from build123d import *

# Parameters (mm, degrees)
SZKIC1_W                    = 40
SZKIC1_H                    = 28
SZKIC1_R                    = 11
DODANIE_WYCI_GNI_CIE1_DEPTH = 10
SZKIC2_W                    = 40
SZKIC2_H                    = 28
DODANIE_WYCI_GNI_CIE2_DEPTH = 3
SFAZOWANIE1_SIZE            = 2
SZKIC3_R                    = 4.3
WYTNIJ_WYCI_GNI_CIE1_DEPTH  = 3
SZKIC4_R                    = 2
WYTNIJ_WYCI_GNI_CIE2_DEPTH  = 6
ZAOKR_GLENIE1_SIZE          = 14
ZAOKR_GLENIE1_SIZE_2        = 8
ZAOKR_GLENIE2_SIZE          = 14
ZAOKR_GLENIE2_SIZE_2        = 8
SZKIC5_R                    = 2.6
WYTNIJ_WYCI_GNI_CIE3_DEPTH  = 7


with BuildPart() as part:
    # Szkic1 → Dodanie-wyciągnięcie1 (new body)
    with BuildSketch(Plane.XY):
        Rectangle(SZKIC1_W, SZKIC1_H)
        Circle(SZKIC1_R, mode=Mode.SUBTRACT)
    extrude(amount=DODANIE_WYCI_GNI_CIE1_DEPTH)

    # Szkic2 → Dodanie-wyciągnięcie2 (add)
    with BuildSketch(Plane(origin=(0, 0, 0), x_dir=(-1, 0, 0), z_dir=(0, 0, -1))):
        Rectangle(SZKIC2_W, SZKIC2_H)
    extrude(amount=DODANIE_WYCI_GNI_CIE2_DEPTH)

    # Sfazowanie1
    sfazowanie1_edges = [part.edges().sort_by_distance(p)[0] for p in [
        (-11, 0, 0),
    ]]
    chamfer(sfazowanie1_edges, length=SFAZOWANIE1_SIZE)

    # Szkic3 → Wytnij-wyciągnięcie1 (cut)
    with BuildSketch(Plane.XY):
        Circle(SZKIC3_R)
    extrude(amount=-WYTNIJ_WYCI_GNI_CIE1_DEPTH, mode=Mode.SUBTRACT)

    # Szkic4 → Wytnij-wyciągnięcie2 (cut)
    with BuildSketch(Plane.XY.offset(10)):
        with Locations((-15, 0)):
            Circle(SZKIC4_R)
        with Locations((15, 0)):
            Circle(SZKIC4_R)
    extrude(amount=-WYTNIJ_WYCI_GNI_CIE2_DEPTH, mode=Mode.SUBTRACT)

    # Zaokrąglenie1
    # an asymmetric fillet: 14, 8 mm, written as the material it takes off along each edge
    with BuildSketch(Plane(origin=(20, -14, -38), x_dir=(-1, 0, 0), z_dir=(0, 0, 1))) as zaokr_glenie1_piece_1:
        with BuildLine():
            Bezier((ZAOKR_GLENIE1_SIZE, 0), (0, 0), (0, -ZAOKR_GLENIE1_SIZE_2), weights=[1, 0.707106781, 1])
            Line((0, -ZAOKR_GLENIE1_SIZE_2), (0, 0))
            Line((0, 0), (ZAOKR_GLENIE1_SIZE, 0))
        make_face()
    extrude(amount=83, mode=Mode.SUBTRACT)
    with BuildSketch(Plane(origin=(-20, 14, 45), x_dir=(0, -1, 0), z_dir=(0, 0, -1))) as zaokr_glenie1_piece_2:
        with BuildLine():
            Bezier((ZAOKR_GLENIE1_SIZE_2, 0), (0, 0), (0, -ZAOKR_GLENIE1_SIZE), weights=[1, 0.707106781, 1])
            Line((0, -ZAOKR_GLENIE1_SIZE), (0, 0))
            Line((0, 0), (ZAOKR_GLENIE1_SIZE_2, 0))
        make_face()
    extrude(amount=83, mode=Mode.SUBTRACT)

    # Zaokrąglenie2
    # an asymmetric fillet: 14, 8 mm, written as the material it takes off along each edge
    with BuildSketch(Plane(origin=(20, 14, -38), x_dir=(-1, 0, 0), z_dir=(0, 0, 1))) as zaokr_glenie2_piece_1:
        with BuildLine():
            Bezier((ZAOKR_GLENIE2_SIZE, 0), (0, 0), (0, ZAOKR_GLENIE2_SIZE_2), weights=[1, 0.707106781, 1])
            Line((0, ZAOKR_GLENIE2_SIZE_2), (0, 0))
            Line((0, 0), (ZAOKR_GLENIE2_SIZE, 0))
        make_face()
    extrude(amount=83, mode=Mode.SUBTRACT)
    with BuildSketch(Plane(origin=(-20, -14, 45), x_dir=(1, 0, 0), z_dir=(0, 0, -1))) as zaokr_glenie2_piece_2:
        with BuildLine():
            Bezier((ZAOKR_GLENIE2_SIZE, 0), (0, 0), (0, -ZAOKR_GLENIE2_SIZE_2), weights=[1, 0.707106781, 1])
            Line((0, -ZAOKR_GLENIE2_SIZE_2), (0, 0))
            Line((0, 0), (ZAOKR_GLENIE2_SIZE, 0))
        make_face()
    extrude(amount=83, mode=Mode.SUBTRACT)

    # Szkic5 → Wytnij-wyciągnięcie3 (cut)
    with BuildSketch(Plane(origin=(0, 0, -3), x_dir=(-1, 0, 0), z_dir=(0, 0, -1))):
        with Locations((-15, 0)):
            Circle(SZKIC5_R)
        with Locations((15, 0)):
            Circle(SZKIC5_R)
    extrude(amount=-WYTNIJ_WYCI_GNI_CIE3_DEPTH, mode=Mode.SUBTRACT)


solid = part.part
The model under review builds one solid part; all positions refer to its coordinate system, in mm. A direction names the side the tool comes from. Round coordinates to 2 decimals unless told otherwise and drop trailing zeros. Loops run counter-clockwise (first coordinate to the right, second up) from the corner with the lowest first, then second, coordinate; pieces in that order, holes last. Notation, with made-up numbers: M -6,34 L 0,34 A19 cw 0,43 Z; hole C -30,41.5 d7. An arc over 180 degrees is marked long. Answer as CSV lines item,"result". Start each with the question number.
Item 1: Wall thickness on line 1 (X direction, y = -0.25, z = 9.75); line 2 (X direction, y = 1.75, z = 1); line 3 (Y direction, x = 4.5, z = 7.75): over which ranges is each line inside the solid? List them lowest first. Write a range as [from, to].
Item 2: For faces 1 (the face through (14, -2, 4)), 2 (the face through (-2.38, -10.74, 5.94)), 3 (the face through (-9.2, 6.4, 10)), list the 3-axis set-ups (+Z, -Z, +X, -X, +Y, -Y) from which the entire face can be reached by the end or side of a thin tool; tool diameter is ignored.
Item 3: Mouldability with a two-part tool opening along Y and no side actions: class faces 4 (the face through (5, 0, -3)), 5 (the face through (-16.6, -1.2, 7)), 6 (the face through (-2, -4, 0)), 7 (the face through (0, 14, 4)) as released by +Y, released by -Y, zero draft, split by the parting line, or undercut.
Item 4: Consider section A-A (x = 0). Write out the cut boundary in (y, z).
Item 5: Insertion check: P1, Ø2, axis at x = -14.5, z = 3, coming from the -Y side; P2, Ø2, axis at x = 13.5, z = 1, coming from the +Y side; P3, Ø6, axis at x = 6.5, y = -4.5, coming from the +Z side. Each pin has a flat end and moves straight along its axis. Give the tip position at first contact, or say it passes through.
Item 6: Consider section B-B (y = 0). State how many separate pieces and enclosed holes the cut face has, then the cut area to 3 significant figures.
Answer:
1,line 1,"x = [-20, -16.98], [-13.02, -11], [11, 13.02], [16.98, 20]"
1,line 2,"x = [-20, -16.92], [-13.08, -9.85], [9.85, 13.08], [16.92, 20]"
1,line 3,"y = [-14, -10.04], [10.04, 14]"
2,face 1,"-Z"
2,face 2,"+Z"
2,face 3,"+Z, +X, -X, +Y, -Y"
3,face 4,"zero draft"
3,face 5,"undercut"
3,face 6,"undercut"
3,face 7,"released by +Y"
4,outline,"M -14,-3 L -4.3,-3 L -4.3,0 L -9,0 L -11,2 L -11,10 L -14,10 Z; M 4.3,-3 L 14,-3 L 14,10 L 11,10 L 11,2 L 9,0 L 4.3,0 Z"
5,P1,"stops at y = -12.76"
5,P2,"stops at y = 13.09"
5,P3,"stops at z = 1.91"
6,separate pieces,"4"
6,enclosed holes,"0"
6,area,"157 mm^2"
